Could you check a few things on this model? Use its own coordinates, in mm. A direction names the side the tool comes from. Round coordinates to 2 decimals unless told otherwise and drop trailing zeros. Order: outer loops, then holes, each group sorted by start corner. A loop starts at its lowest first (then second) coordinate and runs counter-clockwise, first axis right, second up. Notation, with made-up numbers: (41.25, 44) - (56.25, 44) arc R11 cw to (56.25, 63) - close; hole circle Ø7 at (70, 76). An arc over 180 degrees is marked (long way). Use one line per item in the form item = value.
from build123d import *

# Parameters (mm, degrees)
SKETCH_1_W          = 15
SKETCH_1_H          = 10
SKETCH_1_W_2        = 13
SKETCH_1_H_2        = 8
EXTRUDE_1_DEPTH     = 40
CUT_EXTRUDE_1_REACH = 45.875
SKETCH_3_R          = 1.5
CUT_EXTRUDE_2_REACH = 45.875
SKETCH_4_R          = 2


with BuildPart() as part:
    # ｽｹｯﾁ1 → 押し出し-薄板1 (new body)
    with BuildSketch(Plane(origin=(0, 0, 0), x_dir=(1, 0, 0), z_dir=(0, 1, 0))):
        with Locations((7.5, 5)):
            Rectangle(SKETCH_1_W, SKETCH_1_H)
        with Locations((7.5, 5)):
            Rectangle(SKETCH_1_W_2, SKETCH_1_H_2, mode=Mode.SUBTRACT)
    extrude(amount=EXTRUDE_1_DEPTH)

    # ｶｯﾄ - 押し出し1: up to this face of the body (flat: up to its plane)
    cut_extrude_1_end = Plane(part.part.faces().sort_by_distance((0, 20, -5))[0])
    # ｽｹｯﾁ3 → ｶｯﾄ - 押し出し1 (cut, up to the picked face)
    with BuildSketch(Plane(origin=(15, 0, 0), x_dir=(0, 0, -1), z_dir=(1, 0, 0)), mode=Mode.PRIVATE) as cut_extrude_1_sk1:
        with Locations((5, 25)):
            Circle(SKETCH_3_R)
    cut_extrude_1_tool1 = split(extrude(cut_extrude_1_sk1.sketch, amount=-CUT_EXTRUDE_1_REACH, mode=Mode.PRIVATE), bisect_by=cut_extrude_1_end, keep=Keep.BOTH, mode=Mode.PRIVATE)
    # ｽｹｯﾁ3 → ｶｯﾄ - 押し出し1 (cut, up to the picked face)
    with BuildSketch(Plane(origin=(15, 0, 0), x_dir=(0, 0, -1), z_dir=(1, 0, 0)), mode=Mode.PRIVATE) as cut_extrude_1_sk2:
        with Locations((5, 15)):
            Circle(SKETCH_3_R)
    cut_extrude_1_tool2 = split(extrude(cut_extrude_1_sk2.sketch, amount=-CUT_EXTRUDE_1_REACH, mode=Mode.PRIVATE), bisect_by=cut_extrude_1_end, keep=Keep.BOTH, mode=Mode.PRIVATE)
    add(cut_extrude_1_tool1.solids().sort_by(Axis((15, 25, -5), (-1, 0, 0)))[0], mode=Mode.SUBTRACT)
    add(cut_extrude_1_tool2.solids().sort_by(Axis((15, 15, -5), (-1, 0, 0)))[0], mode=Mode.SUBTRACT)

    # ｶｯﾄ - 押し出し2: up to this face of the body (flat: up to its plane)
    cut_extrude_2_end = Plane(part.part.faces().sort_by_distance((7.5, 20, -10))[0])
    # ｽｹｯﾁ4 → ｶｯﾄ - 押し出し2 (cut, up to the picked face)
    with BuildSketch(Plane.XY, mode=Mode.PRIVATE) as cut_extrude_2_sk1:
        with Locations((7.5, 35)):
            Circle(SKETCH_4_R)
    cut_extrude_2_tool1 = split(extrude(cut_extrude_2_sk1.sketch, amount=-CUT_EXTRUDE_2_REACH, mode=Mode.PRIVATE), bisect_by=cut_extrude_2_end, keep=Keep.BOTH, mode=Mode.PRIVATE)
    # ｽｹｯﾁ4 → ｶｯﾄ - 押し出し2 (cut, up to the picked face)
    with BuildSketch(Plane.XY, mode=Mode.PRIVATE) as cut_extrude_2_sk2:
        with Locations((7.5, 5)):
            Circle(SKETCH_4_R)
    cut_extrude_2_tool2 = split(extrude(cut_extrude_2_sk2.sketch, amount=-CUT_EXTRUDE_2_REACH, mode=Mode.PRIVATE), bisect_by=cut_extrude_2_end, keep=Keep.BOTH, mode=Mode.PRIVATE)
    add(cut_extrude_2_tool1.solids().sort_by(Axis((7.5, 35, 0), (0, 0, -1)))[0], mode=Mode.SUBTRACT)
    add(cut_extrude_2_tool2.solids().sort_by(Axis((7.5, 5, 0), (0, 0, -1)))[0], mode=Mode.SUBTRACT)


solid = part.part
Item 1: If we mould it in two halves opening along Z, with no side actions, what happens to faces 1 (the face through (1, 20, -5)), 2 (the face through (5.502, 5.088, -0.493)), 3 (the face through (7, 20, 0)), 4 (the face through (0.507, 26.487, -4.805))? For each: released by +Z, released by -Z, zero draft, split by the parting line, or undercut.
Found:
face_1 = undercut
face_2 = zero draft
face_3 = released by +Z
face_4 = undercut
Item 2: Imagine slicing it at D-D on y = 5. Please give me the cut outline in (x, z).
Found:
outline = (0, -10) - (5.5, -10) - (5.5, -9) - (1, -9) - (1, -1) - (5.5, -1) - (5.5, 0) - (0, 0) - close; (9.5, -10) - (15, -10) - (15, 0) - (9.5, 0) - (9.5, -1) - (14, -1) - (14, -9) - (9.5, -9) - close
Item 3: Imagine slicing it at C-C on z = -7. Please give me the cut outline in (x, y).
Found:
outline = (0, 0) - (1, 0) - (1, 40) - (0, 40) - close; (14, 0) - (15, 0) - (15, 40) - (14, 40) - close
Item 4: I need wall thicknesses on L1, parallel to Y at x = 14.45, z = -5; L2, parallel to Z at x = 11.5, y = 17.5; L3, parallel to X at y = 17.5, z = -6.75. Which ranges of each line are inside material? Lowest first, please.
Found:
L1 = 0 to 13.5, 16.5 to 23.5, 26.5 to 40
L2 = -10 to -9, -1 to 0
L3 = 0 to 1, 14 to 15
Item 5: For faces 5 (the face through (14, 20, -5)), 6 (the face through (7, 20, -10)), which set-ups out of +Z, -Z, +X, -X, +Y, -Y let a thin tool reach every point of the face, with its end or its side?
Found:
face_5 = +Y, -Y
face_6 = -Z, +X, -X, +Y, -Y
Item 6: Imagine slicing it at A-A on z = -5. Please give me the cut outline in (x, y), plus the area to 3 significant figures.
Found:
outline = (0, 0) - (1, 0) - (1, 13.5) - (0, 13.5) - close; (0, 16.5) - (1, 16.5) - (1, 23.5) - (0, 23.5) - close; (0, 26.5) - (1, 26.5) - (1, 40) - (0, 40) - close; (14, 0) - (15, 0) - (15, 13.5) - (14, 13.5) - close; (14, 16.5) - (15, 16.5) - (15, 23.5) - (14, 23.5) - close; (14, 26.5) - (15, 26.5) - (15, 40) - (14, 40) - close
area = 68.0 mm2
Item 7: Imagine slicing it at B-B on x = 12. Please give me the cut outline in (y, z).
Found:
outline = (0, -10) - (40, -10) - (40, -9) - (0, -9) - close; (0, -1) - (40, -1) - (40, 0) - (0, 0) - close
